Design review of the part built by this model. Coordinates are the model's own, in mm. A direction names the side the tool comes from. Give positions to 0.01 mm unless a question says otherwise; leave off trailing zeros. Loops run counter-clockwise (first coordinate to the right, second up) from the corner with the lowest first, then second, coordinate; pieces in that order, holes last. Notation, with made-up numbers: (3.25, 32.5) - (54.25, 32.5) arc R34 cw to (54.25, 64.5) - close; hole circle Ø4 at (81, 39.5). An arc over 180 degrees is marked (long way). Write each question's results on one line, items separated by ' | '.
from build123d import *

# Parameters (mm, degrees)
SKETCH_1_R          = 79.5
EXTRUDE_1_DEPTH     = 5
SKETCH_2_R          = 9.9
EXTRUDE_2_DEPTH     = 50
CHAMFER_1_SIZE      = 0.2
CUT_EXTRUDE_1_DEPTH = 50
CHAMFER_2_SIZE      = 0.4


with BuildPart() as part:
    # 草图1 → 凸台-拉伸1 (new body)
    with BuildSketch(Plane(origin=(0, 0, 0), x_dir=(1, 0, 0), z_dir=(0, 1, 0))):
        with Locations(Location((0, 0, 0), (0, 0, 270))):
            Circle(SKETCH_1_R)
    extrude(amount=EXTRUDE_1_DEPTH)

    # 草图2 → 凸台-拉伸2 (add)
    with BuildSketch(Plane(origin=(0, 0, 0), x_dir=(-1, 0, 0), z_dir=(0, -1, 0))):
        with Locations(Location((0, 0, 0), (0, 0, 270))):
            Circle(SKETCH_2_R)
    extrude(amount=EXTRUDE_2_DEPTH)

    # 倒角1
    chamfer_1_edges = [part.edges().sort_by_distance(p)[0] for p in [
        (0, 5, -79.5),
    ]]
    chamfer(chamfer_1_edges, length=CHAMFER_1_SIZE)

    # 草图3 → 切除-拉伸1 (cut)
    with BuildSketch(Plane(origin=(0, -50, 0), x_dir=(-1, 0, 0), z_dir=(0, -1, 0))):
        with BuildLine():
            Line((4.835339801, -8.753255909), (-5.365688092, -8.438565713))
            ThreePointArc((-5.365688092, -8.438565713), (-0.308342029, -9.995245129), (4.835339801, -8.753255909))
        make_face()
    extrude(amount=-CUT_EXTRUDE_1_DEPTH, mode=Mode.SUBTRACT)

    # 倒角2
    chamfer_2_edges = [part.edges().sort_by_distance(p)[0] for p in [
        (0.265174145, 0, 8.595910811),
        (0, 0, -79.5),
        (-0.305258609, 0, -9.895292678),
    ]]
    chamfer(chamfer_2_edges, length=CHAMFER_2_SIZE)


solid = part.part
(1) Wall thickness on line 1 along Y through (x, z) = (41, 32); line 2 along Z through (x, y) = (-8.5, -35.5); line 3 along Z through (x, y) = (69, 2.5): over which ranges is each line inside the solid? List them lowest first. Write a range as from..to.
Answers below:
line 1: 0..5 | line 2: -5.08..5.08 | line 3: -39.49..39.49
(2) Insertion check: P1, Ø5, axis at x = -3.5, z = -13.5, coming from the -Y side; P2, Ø10, axis at x = 6.5, y = -28.5, coming from the -Z side. Each pin has a flat end and moves straight along its axis. Give the tip position at first contact, or say it passes through.
Answers below:
P1: y = 0 | P2: z = -9.79
(3) Tool access review of faces 1 (the cylindrical face through (78.823, 2.569, -10.349)), 2 (the cylindrical face through (-0.668, -24.853, -9.877)): name each direction out of +Z, -Z, +X, -X, +Y, -Y from which nothing blocks a thin tool from reaching the whole face with its end or side.
Answers below:
face 1: +Y, -Y | face 2: -Y
(4) Take a section at C-C on y = -41. Give the boundary of the cut face in (x, z), plus the area to 3 significant figures.
Answers below:
outline: (-4.64, 8.75) arc R9.9 ccw (long way) to (5.17, 8.44) - close | area: 299 mm2
(5) Take a section at B-B on x = 0. Give the boundary of the cut face in (y, z), plus the area to 3 significant figures.
Answers below:
outline: (-50, -9.9) - (-0.4, -9.9) - (0, -10.3) - (0, -79.1) - (0.4, -79.5) - (4.8, -79.5) - (5, -79.3) - (5, 79.3) - (4.8, 79.5) - (0.4, 79.5) - (0, 79.1) - (0, 9) - (-0.4, 8.6) - (-50, 8.6) - close | area: 1,720 mm2
(6) Take a section at A-A on z = 0. Give the boundary of the cut face in (x, y), plus the area to 3 significant figures.
Answers below:
outline: (-79.5, 0.4) - (-79.1, 0) - (-10.3, 0) - (-9.9, -0.4) - (-9.9, -50) - (9.9, -50) - (9.9, -0.4) - (10.3, 0) - (79.1, 0) - (79.5, 0.4) - (79.5, 4.8) - (79.3, 5) - (-79.3, 5) - (-79.5, 4.8) - close | area: 1,780 mm2
